Geometry: final body of the model. Coordinates: model frame, mm. A direction names the side the tool comes from. Give positions to 0.01 mm unless a question says otherwise; leave off trailing zeros. Write each loop counter-clockwise with the first axis right and the second up, starting at its lowest first coordinate (ties: lowest second). Pieces come first, ordered by that corner, then holes. Notation, with made-up numbers: (-32, -37) -> (19, -37) arc R20 ccw to (19, -9) -> close; hole circle Ø7 at (-13.75, 88.5). An arc over 180 degrees is marked (long way). Answer as a JSON object with one key per item and string values.
from build123d import *

# Parameters (mm, degrees)
SKETCH1_W               = 8
SKETCH1_H               = 8
BOSS_EXTRUDE1_DEPTH     = 3
CUT_EXTRUDE1_DEPTH      = 12.704699911
CUT_EXTRUDE1_DEPTH_BACK = 12.704699911
CUT_EXTRUDE2_DEPTH      = 11
SKETCH4_R               = 1.8
CUT_EXTRUDE3_DEPTH      = 0.8
SKETCH5_W               = 8
SKETCH5_H               = 1
BOSS_EXTRUDE2_DEPTH     = 2
FILLET1_R               = 4
CUT_EXTRUDE4_DEPTH      = 0.4


with BuildPart() as part:
    # Sketch1 → Boss-Extrude1 (new body)
    with BuildSketch(Plane(origin=(0, 0, 0), x_dir=(1, 0, 0), z_dir=(0, 1, 0))):
        with Locations((4, 4)):
            Rectangle(SKETCH1_W, SKETCH1_H)
    extrude(amount=BOSS_EXTRUDE1_DEPTH)

    # Sketch2 → Cut-Extrude1 (cut, two sides: drawn at the far end of the back side and taken through both)
    with BuildSketch(Plane.XY.offset(-CUT_EXTRUDE1_DEPTH_BACK)):
        Polygon((0, 0), (0.6, 3), (0, 3), align=None)
        Polygon((8, 0), (7.4, 3), (8, 3), align=None)
    extrude(amount=CUT_EXTRUDE1_DEPTH + CUT_EXTRUDE1_DEPTH_BACK, mode=Mode.SUBTRACT)

    # Sketch3 → Cut-Extrude2 (cut)
    with BuildSketch(Plane(origin=(0, 0, 0), x_dir=(0, 0, -1), z_dir=(1, 0, 0))):
        Polygon((0, 0), (0.6, 3), (0, 3), align=None)
        Polygon((8, 3), (7.4, 3), (8, 0), align=None)
    extrude(amount=CUT_EXTRUDE2_DEPTH, mode=Mode.SUBTRACT)

    # Sketch4 → Cut-Extrude3 (cut)
    with BuildSketch(Plane.XZ):
        with Locations(Location((4, -3.75, 0), (0, 0, 270))):
            Circle(SKETCH4_R)
    extrude(amount=-CUT_EXTRUDE3_DEPTH, mode=Mode.SUBTRACT)

    # Sketch5 → Boss-Extrude2 (add)
    with BuildSketch(Plane.XZ):
        with Locations((4, -7.5)):
            Rectangle(SKETCH5_W, SKETCH5_H)
    extrude(amount=BOSS_EXTRUDE2_DEPTH)

    # Fillet1
    # the kernel refuses this fillet: 4 mm, written as the material it takes off along each edge
    with BuildSketch(Plane(origin=(8, -2, -16.660254038), x_dir=(0, 1, 0), z_dir=(0, 0, 1)), Plane(origin=(0, -2, 1.660254038), x_dir=(0, 1, 0), z_dir=(0, 0, -1))) as fillet1_piece_1:
        with BuildLine():
            CenterArc((4, 3.464101615), FILLET1_R, 180, 60)
            Line((0, 3.464101615), (-0.08, 3.464101615))
            Line((-0.08, 3.464101615), (-0.08, 0))
            Line((-0.08, 0), (0, -0.08))
            ThreePointArc((0, -0.08), (1, -0.08), (1.96, -0.069282032))
            Line((1.96, -0.069282032), (2, 0))
        make_face()
    extrude(amount=18.320508076, mode=Mode.SUBTRACT)

    # Sketch6 → Cut-Extrude4 (cut)
    with BuildSketch(Plane(origin=(0, 3, 0), x_dir=(1, 0, 0), z_dir=(0, 1, 0))):
        with BuildLine():
            Line((2.436272881, 5.979723732), (3.903420317, 5.979723732))
            add(Edge.make_bspline(
                [(3.903420317, 5.979723732), (3.943490496, 5.979744505), (4.021516441, 5.979784954), (4.134752515, 5.975087302), (4.240642802, 5.970362082), (4.338883372, 5.960903224), (4.429815049, 5.950988663), (4.51360101, 5.938436084), (4.589711972, 5.922348579), (4.637707501, 5.909661658), (4.660631856, 5.903601937)],
                knots=[0, 0, 0, 0, 1.259756885, 2.453039283, 3.563158368, 4.591894114, 5.55549294, 6.43918076, 7.254497783, 8, 8, 8, 8], degree=3))
            add(Edge.make_bspline(
                [(4.660631856, 5.903601937), (4.689300162, 5.894258489), (4.74612039, 5.87573989), (4.829420592, 5.843292221), (4.908343197, 5.803050568), (4.985816138, 5.760749105), (5.058380803, 5.710732544), (5.129877456, 5.658697008), (5.195666079, 5.598419283), (5.281939397, 5.514177193), (5.380383811, 5.396825298), (5.483519335, 5.241163905), (5.570813292, 5.070304112), (5.630456537, 4.917219685), (5.670729972, 4.787084992), (5.697056277, 4.682749965), (5.719418871, 4.572846322), (5.737778631, 4.457346355), (5.752043635, 4.336250048), (5.762664083, 4.209589679), (5.767837312, 4.07725583), (5.769008616, 3.987205692), (5.769606215, 3.941262194)],
                knots=[0, 0, 0, 0, 0.745524535, 1.477620414, 2.207090574, 2.934465325, 3.657932502, 4.384347339, 5.118673636, 5.861150177, 7.365375624, 8.894729774, 10.468936425, 12.099947606, 12.950091786, 13.83580991, 14.759228729, 15.722225242, 16.726454549, 17.773376212, 18.863978586, 20, 20, 20, 20], degree=3))
            add(Edge.make_bspline(
                [(5.769606215, 3.941262194), (5.768515323, 3.861857727), (5.766405561, 3.708291084), (5.741963835, 3.486695058), (5.70674022, 3.280872561), (5.667035899, 3.152471539), (5.647811343, 3.090300655)],
                knots=[0, 0, 0, 0, 1.103207939, 2.133582005, 3.096293362, 4, 4, 4, 4], degree=3))
            add(Edge.make_bspline(
                [(5.647811343, 3.090300655), (5.635116766, 3.054625647), (5.610144552, 2.98444734), (5.566445051, 2.883214788), (5.519227431, 2.786877042), (5.468100041, 2.695510004), (5.412804571, 2.609524646), (5.353134197, 2.529178156), (5.290013855, 2.453412746), (5.244286819, 2.406778778), (5.221529292, 2.383569886)],
                knots=[0, 0, 0, 0, 1.090884612, 2.145940218, 3.175104604, 4.181306866, 5.161203701, 6.118658341, 7.063689906, 8, 8, 8, 8], degree=3))
            add(Edge.make_bspline(
                [(5.221529292, 2.383569886), (5.184702113, 2.350450915), (5.108759222, 2.282154876), (4.974934842, 2.197635799), (4.823675662, 2.122952418), (4.714264019, 2.084588805), (4.657426727, 2.06465963)],
                knots=[0, 0, 0, 0, 0.908140292, 1.872714733, 2.8949153, 4, 4, 4, 4], degree=3))
            add(Edge.make_bspline(
                [(4.657426727, 2.06465963), (4.634546833, 2.057632533), (4.587060796, 2.043048157), (4.511767003, 2.027471741), (4.431388989, 2.011061834), (4.344999886, 2.001176252), (4.253496453, 1.990751469), (4.156149493, 1.984898536), (4.053296456, 1.980743294), (3.98275208, 1.980068625), (3.946689548, 1.979723732)],
                knots=[0, 0, 0, 0, 0.799129865, 1.658552685, 2.566799617, 3.538529252, 4.561352959, 5.643373779, 6.795284424, 8, 8, 8, 8], degree=3))
            Line((3.946689548, 1.979723732), (2.436272881, 1.979723732))
            Line((2.436272881, 1.979723732), (2.436272881, 5.979723732))
        make_face()
        with BuildLine():
            Line((3.205503651, 5.313057065), (3.205503651, 2.646390399))
            Line((3.205503651, 2.646390399), (3.838516471, 2.646390399))
            add(Edge.make_bspline(
                [(3.838516471, 2.646390399), (3.86709534, 2.646617049), (3.922120581, 2.647053436), (4.001743514, 2.648335709), (4.07491632, 2.651807064), (4.142022322, 2.655402822), (4.202886818, 2.661343643), (4.257774639, 2.667186667), (4.306380252, 2.675360935), (4.336400272, 2.681813595), (4.350535702, 2.684851937)],
                knots=[0, 0, 0, 0, 1.333384787, 2.567275092, 3.714769766, 4.750907381, 5.701951617, 6.567520054, 7.325492842, 8, 8, 8, 8], degree=3))
            add(Edge.make_bspline(
                [(4.350535702, 2.684851937), (4.38364248, 2.693686468), (4.44812575, 2.710893803), (4.538666782, 2.749253907), (4.62059475, 2.795531175), (4.695281698, 2.8511776), (4.762590099, 2.92150181), (4.820046047, 3.011440962), (4.873220012, 3.118706088), (4.909633556, 3.221385639), (4.935771128, 3.313096613), (4.95346412, 3.390071897), (4.967446413, 3.47335137), (4.979473009, 3.562606359), (4.989190784, 3.657722085), (4.995237644, 3.759042029), (4.999364663, 3.866442163), (5.000032135, 3.940189623), (5.000375445, 3.978121168)],
                knots=[0, 0, 0, 0, 1.038686998, 2.023088296, 2.974059649, 3.888265163, 4.839857954, 5.909819677, 7.113156087, 8.466843969, 9.20827164, 10.006482943, 10.861893492, 11.769681931, 12.739021491, 13.762258324, 14.849031541, 16, 16, 16, 16], degree=3))
            add(Edge.make_bspline(
                [(5.000375445, 3.978121168), (5.000034775, 4.01605283), (4.999374834, 4.089533605), (4.995254144, 4.196132914), (4.989241251, 4.29585735), (4.979454269, 4.38883019), (4.967614104, 4.475179926), (4.953468032, 4.554979633), (4.935881696, 4.627705609), (4.909721893, 4.71410541), (4.870064977, 4.811221472), (4.816099655, 4.917402921), (4.749828382, 5.00790436), (4.676605078, 5.08652444), (4.592177372, 5.151224792), (4.498716105, 5.205415106), (4.394186359, 5.247475499), (4.319831067, 5.2653904), (4.281625445, 5.274595527)],
                knots=[0, 0, 0, 0, 1.117996097, 2.165769068, 3.143980016, 4.062055362, 4.920439205, 5.712587309, 6.449616741, 7.124491204, 8.371470382, 9.537068822, 10.625202851, 11.666538334, 12.693249444, 13.747832046, 14.842779399, 16, 16, 16, 16], degree=3))
            add(Edge.make_bspline(
                [(4.281625445, 5.274595527), (4.265088191, 5.27766838), (4.228679487, 5.284433627), (4.168262747, 5.292335475), (4.097380449, 5.298199321), (4.015671249, 5.304185793), (3.923465993, 5.307602683), (3.820378875, 5.311168762), (3.706841263, 5.312386928), (3.627511913, 5.312827267), (3.586112625, 5.313057065)],
                knots=[0, 0, 0, 0, 0.578738571, 1.274160813, 2.095454135, 3.025967819, 4.093109015, 5.270126069, 6.575371698, 8, 8, 8, 8], degree=3))
            Line((3.586112625, 5.313057065), (3.205503651, 5.313057065))
        make_face(mode=Mode.SUBTRACT)
    extrude(amount=-CUT_EXTRUDE4_DEPTH, mode=Mode.SUBTRACT)


solid = part.part
Q1. Set-up query: faces 4 (the flat face through (3, 0, -2)), 5 (the flat face through (4, -2, -7.5)), 6 (the flat face through (4, 0.8, -4)). Return all of +Z, -Z, +X, -X, +Y, -Y with unobstructed straight access to the full face (end or side cutting, diameter ignored); none if empty.
Values:
{"face 4": "+Z, +X, -X, -Y", "face 5": "+Z, -Z, +X, -X, -Y", "face 6": "-Y"}
Q2. Material intervals for L1, parallel to Y at x = 5.75, z = -6.25; L2, parallel to Z at x = 4, y = -0.25; L3, parallel to Y at x = 2.5, z = -4.5, sorted ascending. Write a range as from..to.
Values:
{"L1": "0..3", "L2": "-8..-7", "L3": "0.8..2.6"}
Q3. Cut plane D-D (x = 6.5). Return the cut outline in (y, z), and give its area (3 significant figures).
Values:
{"outline": "(-1.48, -8) -> (0, -8) -> (3, -7.4) -> (3, -0.6) -> (0, 0) -> (0, -7) -> (-1.48, -7) -> close", "area": "23.7 mm²"}
Q4. First-contact query: P1, Ø3, axis at x = 4, z = -2.5, coming from the -Y side; P2, Ø0.6, axis at x = 5.5, y = -1.5, coming from the +Z side. Flat tips, straight axial feed; report the tip coordinate or a pass-through.
Values:
{"P1": "y = 0", "P2": "z = -7"}
Q5. Cut plane B-B (y = 2.05). Return the cut outline in (x, z).
Values:
{"outline": "(0.41, -7.59) -> (7.59, -7.59) -> (7.59, -0.41) -> (0.41, -0.41) -> close"}
Q6. Cut plane A-A (x = 7.75). Return the cut outline in (y, z), and give its area (3 significant figures).
Values:
{"outline": "(-0.38, -8) -> (0, -8) -> (1.25, -7.75) -> (1.25, -0.25) -> (0, 0) -> (0, -7) -> (-0.38, -7) -> close", "area": "10.1 mm²"}
Q7. Mould query, pull axis X, two halves, no side actions, for faces 1 (the cylindrical face through (6.51, -1.48, -7.51)), 2 (the flat face through (3.9, 1.5, -0.3)), 3 (the flat face through (3, 2.6, -4)). Classes: pulls with the +X half, pulls with the -X half, needs draft (parallel to the pull), parting line crosses it, or undercut.
Values:
{"face 1": "pulls with the +X half", "face 2": "needs draft", "face 3": "undercut"}
Q8. Cut plane C-C (z = -6.25). Return the cut outline in (x, y), and give its area (3 significant figures).
Values:
{"outline": "(0, 0) -> (8, 0) -> (7.4, 3) -> (0.6, 3) -> close", "area": "22.2 mm²"}
